Could you check a few things on this model? Use its own coordinates, in mm. Face numbers are marked on the shaded views. A direction names the side the tool comes from. Coordinates: 2 decimals unless noted, no trailing zeros. Order: outer loops, then holes, each group sorted by start corner. A loop starts at its lowest first (then second) coordinate and runs counter-clockwise, first axis right, second up. Notation, with made-up numbers: (5, 4) -> (23, 4) arc R29 ccw to (23, 41) -> close; hole circle Ø4 at (46, 7). An arc over 180 degrees is marked (long way). Put each result on its own line as item: value. Start each with the question number.
Q1. Please list where these lines run through material, in increasing order: line 1 along X through (y, z) = (1.75, -1.7); line 2 along Z through (x, y) = (-0.1, 3.25).
Q2. If we section it at A-A (x = 1.3): Please give me the cut outline in (y, z).
Q3. Will these pins go through, and if not, where does the flat tip stop? pin 1 (0.5 mm diameter, centred on x = -2, y = -3, fed in from +Z); pin 2 (1.1 mm diameter, centred on y = 1, z = 2, fed in from +X); pin 3 (1.1 mm diameter, centred on x = -2, y = 0.5, fed in from -Z).
Q4. If we section it at B-B (y = 6.75): Please give me the cut outline in (x, z), and give its area (3 significant figures).
Q5. If we section it at C-C (z = -1.75): Please give me the cut outline in (x, y).
Q6. For the marked faces 1, 2 and 3, which set-ups out of +Z, -Z, +X, -X, +Y, -Y let a thin tool reach every point of the face, with its end or its side?
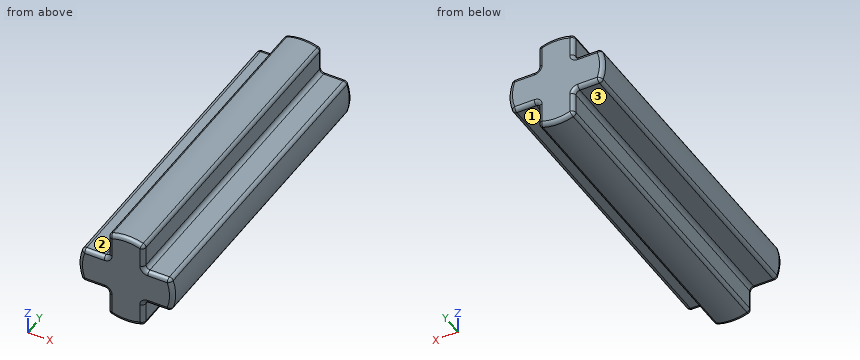
from build123d import *

# Parameters (mm, degrees)
BOSS_EXTRUDE1_DEPTH = 8
FILLET3_R           = 0.2


with BuildPart() as part:
    # Sketch1 → Boss-Extrude1 (new, symmetric)
    with BuildSketch(Plane(origin=(0, 0, 0), x_dir=(1, 0, 0), z_dir=(0, 1, 0))):
        with BuildLine():
            Line((-0.9, -0.9), (-0.9, -2.224859546))
            ThreePointArc((-0.9, -2.224859546), (0, -2.4), (0.9, -2.224859546))
            Line((0.9, -2.224859546), (0.9, -0.9))
            Line((0.9, -0.9), (2.224859546, -0.9))
            ThreePointArc((2.224859546, -0.9), (2.4, 0), (2.224859546, 0.9))
            Line((2.224859546, 0.9), (0.9, 0.9))
            Line((0.9, 0.9), (0.9, 2.224859546))
            ThreePointArc((0.9, 2.224859546), (0, 2.4), (-0.9, 2.224859546))
            Line((-0.9, 2.224859546), (-0.9, 0.9))
            Line((-0.9, 0.9), (-2.224859546, 0.9))
            ThreePointArc((-2.224859546, 0.9), (-2.4, 0), (-2.224859546, -0.9))
            Line((-2.224859546, -0.9), (-0.9, -0.9))
        make_face()
    extrude(amount=BOSS_EXTRUDE1_DEPTH, both=True)

    # Fillet3
    fillet3_edges = [part.edges().sort_by_distance(p)[0] for p in [
        (-1.562429773, -8, -0.9),
        (-0.9, -8, -1.562429773),
        (-0.9, 8, 1.562429773),
        (0, -8, -2.4),
        (0.9, -8, -1.562429773),
        (1.562429773, -8, -0.9),
        (2.4, -8, 0),
        (1.562429773, -8, 0.9),
        (0.9, -8, 1.562429773),
        (0, -8, 2.4),
        (-0.9, -8, 1.562429773),
        (-1.562429773, -8, 0.9),
        (-2.4, -8, 0),
        (0, 8, 2.4),
        (-2.224859546, 0, -0.9),
        (-0.9, 0, -0.9),
        (-0.9, 0, -2.224859546),
        (0.9, 8, 1.562429773),
        (0.9, 0, -2.224859546),
        (0.9, 0, -0.9),
        (2.224859546, 0, -0.9),
        (2.224859546, 0, 0.9),
        (0.9, 0, 0.9),
        (0.9, 0, 2.224859546),
        (-0.9, 0, 2.224859546),
        (-0.9, 0, 0.9),
        (-2.224859546, 0, 0.9),
        (1.562429773, 8, 0.9),
        (2.4, 8, 0),
        (1.562429773, 8, -0.9),
        (0.9, 8, -1.562429773),
        (0, 8, -2.4),
        (-0.9, 8, -1.562429773),
        (-1.562429773, 8, -0.9),
        (-2.4, 8, 0),
        (-1.562429773, 8, 0.9),
    ]]
    fillet(fillet3_edges, radius=FILLET3_R)


solid = part.part
The answers:
1. line 1: -0.9 to 0.9
1. line 2: -2.4 to 2.4
2. outline: (-8, -0.7) arc R0.2 ccw to (-7.8, -0.9) -> (7.8, -0.9) arc R0.2 ccw to (8, -0.7) -> (8, 0.7) arc R0.2 ccw to (7.8, 0.9) -> (-7.8, 0.9) arc R0.2 ccw to (-8, 0.7) -> close
3. pin 1: z = 0.9
3. pin 2: x = 0.9
3. pin 3: z = -0.9
4. outline: (-2.28, -0.76) arc R0.2 ccw to (-2.09, -0.9) -> (-1.1, -0.9) arc R0.2 cw to (-0.9, -1.1) -> (-0.9, -2.09) arc R0.2 ccw to (-0.76, -2.28) arc R2.4 ccw to (0.76, -2.28) arc R0.2 ccw to (0.9, -2.09) -> (0.9, -1.1) arc R0.2 cw to (1.1, -0.9) -> (2.09, -0.9) arc R0.2 ccw to (2.28, -0.76) arc R2.4 ccw to (2.28, 0.76) arc R0.2 ccw to (2.09, 0.9) -> (1.1, 0.9) arc R0.2 cw to (0.9, 1.1) -> (0.9, 2.09) arc R0.2 ccw to (0.76, 2.28) arc R2.4 ccw to (-0.76, 2.28) arc R0.2 ccw to (-0.9, 2.09) -> (-0.9, 1.1) arc R0.2 cw to (-1.1, 0.9) -> (-2.09, 0.9) arc R0.2 ccw to (-2.28, 0.76) arc R2.4 ccw to start
4. area: 13.6 mm^2
5. outline: (-0.9, -7.8) arc R0.2 ccw to (-0.7, -8) -> (0.7, -8) arc R0.2 ccw to (0.9, -7.8) -> (0.9, 7.8) arc R0.2 ccw to (0.7, 8) -> (-0.7, 8) arc R0.2 ccw to (-0.9, 7.8) -> close
6. face 1: -Z, +X, +Y, -Y
6. face 2: +Z, -X, +Y, -Y
6. face 3: -Z, -X, +Y, -Y
